Geometry check sheet. Reference: the model listing, model coordinates, mm. Face numbers are marked on the shaded views. Give positions to 0.01 mm unless a question says otherwise; leave off trailing zeros. Order: outer loops, then holes, each group sorted by start corner. A loop starts at its lowest first (then second) coordinate and runs counter-clockwise, first axis right, second up.
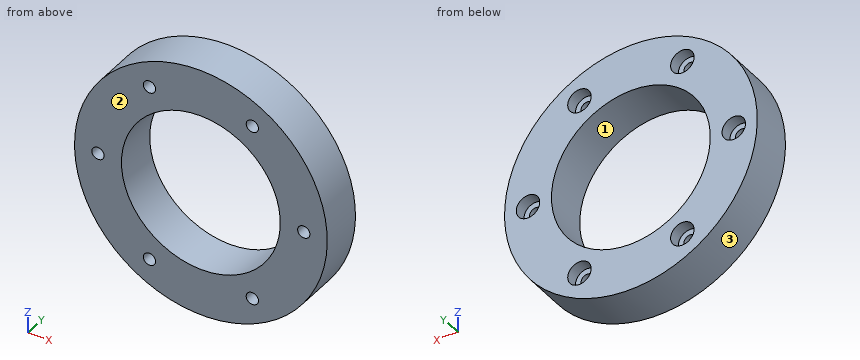
from build123d import *

# Parameters (mm, degrees)
SKETCH_1_R          = 35
SKETCH_1_R_2        = 1.7
SKETCH_1_R_3        = 22
EXTRUDE_1_DEPTH     = 12
SKETCH_2_R          = 3.25
CUT_EXTRUDE_1_DEPTH = 3.3


with BuildPart() as part:
    # 草图1 → 凸台-拉伸1 (new body)
    with BuildSketch(Plane(origin=(0, 0, 0), x_dir=(1, 0, 0), z_dir=(0, 1, 0))):
        with Locations(Location((0, 0, 0), (0, 0, 270))):
            Circle(SKETCH_1_R)
        with Locations(Location((-28.5, 0, 0), (0, 0, 270))):
            Circle(SKETCH_1_R_2, mode=Mode.SUBTRACT)
        with Locations(Location((-14.25, 24.681724008, 0), (0, 0, 270))):
            Circle(SKETCH_1_R_2, mode=Mode.SUBTRACT)
        with Locations(Location((14.25, 24.681724008, 0), (0, 0, 270))):
            Circle(SKETCH_1_R_2, mode=Mode.SUBTRACT)
        with Locations(Location((28.5, 0, 0), (0, 0, 270))):
            Circle(SKETCH_1_R_2, mode=Mode.SUBTRACT)
        with Locations(Location((14.25, -24.681724008, 0), (0, 0, 270))):
            Circle(SKETCH_1_R_2, mode=Mode.SUBTRACT)
        with Locations(Location((-14.25, -24.681724008, 0), (0, 0, 270))):
            Circle(SKETCH_1_R_2, mode=Mode.SUBTRACT)
        with Locations(Location((0, 0, 0), (0, 0, 270))):
            Circle(SKETCH_1_R_3, mode=Mode.SUBTRACT)
    extrude(amount=EXTRUDE_1_DEPTH)

    # 草图2 → 切除-拉伸1 (cut)
    with BuildSketch(Plane(origin=(0, 12, 0), x_dir=(1, 0, 0), z_dir=(0, 1, 0))):
        with Locations(Location((-28.5, 0, 0), (0, 0, 270))):
            Circle(SKETCH_2_R)
        with Locations(Location((-14.25, 24.681724008, 0), (0, 0, 270))):
            Circle(SKETCH_2_R)
        with Locations(Location((14.25, 24.681724008, 0), (0, 0, 270))):
            Circle(SKETCH_2_R)
        with Locations(Location((28.5, 0, 0), (0, 0, 270))):
            Circle(SKETCH_2_R)
        with Locations(Location((14.25, -24.681724008, 0), (0, 0, 270))):
            Circle(SKETCH_2_R)
        with Locations(Location((-14.25, -24.681724008, 0), (0, 0, 270))):
            Circle(SKETCH_2_R)
    extrude(amount=-CUT_EXTRUDE_1_DEPTH, mode=Mode.SUBTRACT)


solid = part.part
Item 1: Sectioned sample at D-D (z = -12.5). Enter the section's corners in (x, y), and give its area (3 significant figures).
Reported:
outline: (-32.69, 0) - (-18.1, 0) - (-18.1, 12) - (-32.69, 12) - close; (18.1, 0) - (32.69, 0) - (32.69, 12) - (18.1, 12) - close
area: 350 mm2
Item 2: Scan lines: L1, parallel to X at y = 6, z = -25.5; L2, parallel to Z at x = 16, y = 9; L3, parallel to X at y = 1, z = -25. Record each from-to range of solid material in increasing order.
Reported:
L1: x = -23.97 to -15.74, -12.76 to 12.76, 15.74 to 23.97
L2: z = -31.13 to -27.42, -21.94 to -15.1, 15.1 to 21.94, 27.42 to 31.13
L3: x = -24.49 to -15.92, -12.58 to 12.58, 15.92 to 24.49
Item 3: Gauge pin test, flat ends, axial feed: pin 1 (2 mm diameter, centred on x = -15, z = -25.5, fed in from +Y); pin 2 (2 mm diameter, centred on x = -18.5, y = 4.5, fed in from -Z); pin 3 (3 mm diameter, centred on x = 12, y = 8.5, fed in from +Z); pin 4 (2 mm diameter, centred on x = -14.25, z = -24.68, fed in from -Y). Record the tip position at first contact, or that the pin passes through.
Reported:
pin 1: stops at y = 8.7
pin 2: stops at z = -30.31
pin 3: stops at z = 33.39
pin 4: passes through
Item 4: Draft check along Z on the marked faces 1, 2 and 3. Enter one of: released by +Z, released by -Z, zero draft, split by the parting line, or undercut.
Reported:
face 1: undercut
face 2: zero draft
face 3: split by the parting line
Item 5: Sectioned sample at B-B (y = 10.25). Enter the section's corners in (x, z).
Reported:
outline: circle Ø70 at (0, 0); hole circle Ø6.5 at (-28.5, 0); hole circle Ø44 at (0, 0); hole circle Ø6.5 at (-14.25, -24.68); hole circle Ø6.5 at (-14.25, 24.68); hole circle Ø6.5 at (14.25, -24.68); hole circle Ø6.5 at (14.25, 24.68); hole circle Ø6.5 at (28.5, 0)
Item 6: Sectioned sample at C-C (x = 0). Enter the section's corners in (y, z), and give its area (3 significant figures).
Reported:
outline: (0, -35) - (12, -35) - (12, -22) - (0, -22) - close; (0, 22) - (12, 22) - (12, 35) - (0, 35) - close
area: 312 mm2
Item 7: Sectioned sample at A-A (z = 0). Enter the section's corners in (x, y), and give its area (3 significant figures).
Reported:
outline: (-35, 0) - (-30.2, 0) - (-30.2, 8.7) - (-31.75, 8.7) - (-31.75, 12) - (-35, 12) - close; (-26.8, 0) - (-22, 0) - (-22, 12) - (-25.25, 12) - (-25.25, 8.7) - (-26.8, 8.7) - close; (22, 0) - (26.8, 0) - (26.8, 8.7) - (25.25, 8.7) - (25.25, 12) - (22, 12) - close; (30.2, 0) - (35, 0) - (35, 12) - (31.75, 12) - (31.75, 8.7) - (30.2, 8.7) - close
area: 210 mm2
